The listing builds one solid part. Answer for the finished solid, in the listing's coordinates (mm). Give positions to 0.01 mm unless a question says otherwise; leave off trailing zeros. Order: outer loops, then holes, each group sorted by start corner. A loop starts at its lowest first (then second) coordinate and runs counter-clockwise, first axis right, second up. Notation, with made-up numbers: (-30, -4) - (1, -4) arc R17 ccw to (1, 26) - close; hole circle Ø7 at (9.25, 32). An arc over 180 degrees is marked (long way). Answer in a Markdown table with one row per item.
from build123d import *

# Parameters (mm, degrees)
F0_R     = 2.38125
F1_DEPTH = 3.175
F2_R     = 6.35
F3_SIZE  = 1.4111111111


with BuildPart() as f1:
    # F0 (on Top) → F1 (new body)
    with BuildSketch(Plane.XY):
        with BuildLine():
            Line((123.3248860695, 4.1671875), (3.6751139305, 4.1671875))
            ThreePointArc((3.6751139305, 4.1671875), (-5.55625, 0), (3.6751139305, -4.1671875))
            Line((3.6751139305, -4.1671875), (123.3248860695, -4.1671875))
            ThreePointArc((123.3248860695, -4.1671875), (132.55625, 0), (123.3248860695, 4.1671875))
        make_face()
        Circle(F0_R, mode=Mode.SUBTRACT)
        with Locations((127, 0)):
            Circle(F0_R, mode=Mode.SUBTRACT)
    extrude(amount=F1_DEPTH)

    # F2
    f2_edges = [f1.edges().sort_by_distance(p)[0] for p in [
        (3.675114, 4.167187, 1.5875),
        (3.675114, -4.167188, 1.5875),
        (123.324886, -4.167187, 1.5875),
        (123.324886, 4.167187, 1.5875),
    ]]
    fillet(f2_edges, radius=F2_R)

    # F3
    f3_edges = [f1.edges().sort_by_distance(p)[0] for p in [
        (63.5, 4.167187, 3.175),
        (63.5, 4.167187, 0),
    ]]
    chamfer(f3_edges, length=F3_SIZE)


solid = f1.part
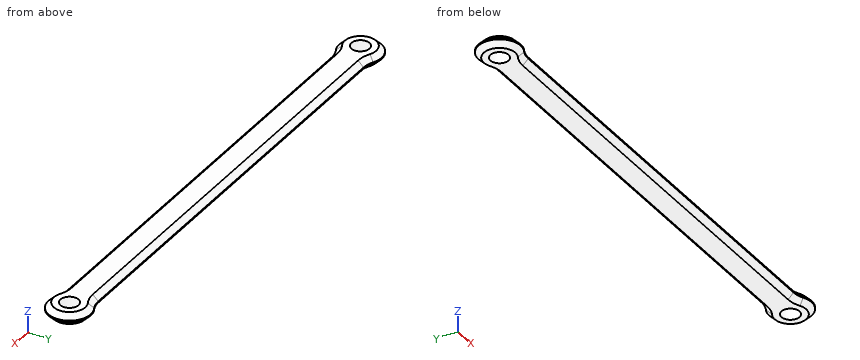
Item 1: Consider line 1 (Y direction, x = 0, z = 2.4); line 2 (X direction, y = 0.75, z = 2.2); line 3 (Y direction, x = 127, z = 1.55). Determine where each line is inside the solid, lowest interval first.
Answer block:
| item | result |
|---|---|
| line 1 | -4.92 to -2.38, 2.38 to 4.92 |
| line 2 | -5.06 to -2.26, 2.26 to 124.74, 129.26 to 132.06 |
| line 3 | -5.56 to -2.38, 2.38 to 5.56 |
Item 2: Find section C-C on x = 29.5. Write down the section's boundary in (y, z) (3 decimals).
Answer block:
| item | result |
|---|---|
| outline | (-4.167, 1.411) - (-2.756, 0) - (2.756, 0) - (4.167, 1.411) - (4.167, 1.764) - (2.756, 3.175) - (-2.756, 3.175) - (-4.167, 1.764) - close |
Item 3: Find section B-B on y = 0. Write down the section's boundary in (x, z) (3 decimals), then the cut area to 3 significant figures.
Answer block:
| item | result |
|---|---|
| outline | (-5.556, 1.411) - (-4.145, 0) - (-2.381, 0) - (-2.381, 3.175) - (-4.145, 3.175) - (-5.556, 1.764) - close; (2.381, 0) - (124.619, 0) - (124.619, 3.175) - (2.381, 3.175) - close; (129.381, 0) - (131.145, 0) - (132.556, 1.411) - (132.556, 1.764) - (131.145, 3.175) - (129.381, 3.175) - close |
| area | 404 mm² |
Item 4: Find section A-A on x = 0. Write down the section's boundary in (y, z) (3 decimals).
Answer block:
| item | result |
|---|---|
| outline | (-5.556, 1.411) - (-4.145, 0) - (-2.381, 0) - (-2.381, 3.175) - (-4.145, 3.175) - (-5.556, 1.764) - close; (2.381, 0) - (4.145, 0) - (5.556, 1.411) - (5.556, 1.764) - (4.145, 3.175) - (2.381, 3.175) - close |
Item 5: Each of these flat-tipped pins is pushed along its axis until it touches: P1, Ø1, axis at y = -0.5, z = 2.5, coming from the +X side; P2, Ø1, axis at x = 117, z = 1.5, coming from the +Y side. Where does it stop, or does it pass through?
Answer block:
| item | result |
|---|---|
| P1 | x = 132.3 |
| P2 | y = 4.17 |
